```python
from build123d import *

# Parameters (mm, degrees)
EXTRUDE_1_DEPTH     = 10
HOLE_WIZARD_1_D     = 3.05
HOLE_WIZARD_1_DEPTH = 14
HOLE_WIZARD_2_D     = 5.01
HOLE_WIZARD_2_DEPTH = 14
HOLE_WIZARD_3_D     = 5.05
HOLE_WIZARD_3_DEPTH = 14
FILLET_1_R          = 2
FILLET_2_R          = 4


with BuildPart() as part:
    # 草图1 → 凸台-拉伸1 (new body)
    with BuildSketch(Plane.XZ):
        with BuildLine():
            Line((-28, -5.5), (-28, -12.193872478))
            ThreePointArc((-28, -12.193872478), (-26.845236523, -14.006488052), (-24.714424781, -13.725961365))
            Line((-24.714424781, -13.725961365), (-13.123475383, -4))
            Line((-13.123475383, -4), (-5.123475383, -4))
            ThreePointArc((-5.123475383, -4), (-0.488094847, -6.481648202), (4.466659496, -4.722176717))
            add(Edge.make_bspline(
                [(20.490071148, 0), (14.378134184, 3.89268165), (4.466659496, -4.722176717)],
                knots=[0.252803303, 0.252803303, 0.252803303, 2.064431363, 2.064431363, 2.064431363], degree=2, weights=[1, 0.617045201, 1]))
            ThreePointArc((20.490071148, 0), (24.593372298, 1.499185377), (22.849655998, 5.50469291))
            add(Edge.make_bspline(
                [(4.159420521, 4.994919512), (11.553776754, 7.153354998), (17.783855246, 7.323279465), (22.849655998, 5.50469291)],
                knots=[0, 0, 0, 0, 1, 1, 1, 1], degree=3))
            ThreePointArc((4.159420521, 4.994919512), (-0.692687991, 6.462985637), (-5.123475383, 4))
            Line((-5.123475383, 4), (-28.225082782, 4))
            ThreePointArc((-28.225082782, 4), (-37.111262075, 2.031009601), (-32, -5.5))
            Line((-32, -5.5), (-28, -5.5))
        make_face()
    extrude(amount=-EXTRUDE_1_DEPTH)

    # 草图2 → 旋转1 (revolve)
    with BuildSketch(Plane(origin=(0, 0, 0), x_dir=(-1, 0, 0), z_dir=(0, 0, -1)), mode=Mode.PRIVATE) as revolve_1_sk:
        Polygon((-3.99, -4), (0, -4), (0, 0), (-5, 0), (-5, -0.5), (-3.99, -0.5), align=None)
    revolve(revolve_1_sk.sketch.rotate(Axis((0, -4, 0), (0, 1, 0)), 270), axis=Axis((0, -4, 0), (0, 1, 0)))

    # 草图3 → 旋转2 (revolve)
    with BuildSketch(Plane.XY, mode=Mode.PRIVATE) as revolve_2_sk:
        Polygon((3.99, 14), (0, 14), (0, 10), (5, 10), (5, 10.5), (3.99, 10.5), align=None)
    revolve(revolve_2_sk.sketch.rotate(Axis((0, 14, 0), (0, -1, 0)), 270), axis=Axis((0, 14, 0), (0, -1, 0)))

    # 孔1
    with Locations(Plane(origin=(0, 10, 0), x_dir=(1, 0, 0), z_dir=(0, 1, 0))):
        with Locations((21.836015336, -2.681125555)):
            Hole(HOLE_WIZARD_1_D / 2, depth=HOLE_WIZARD_1_DEPTH)

    # 孔2
    with Locations(Plane(origin=(0, 10, 0), x_dir=(1, 0, 0), z_dir=(0, 1, 0))):
        with Locations((-23.339745962, 5)):
            Hole(HOLE_WIZARD_2_D / 2, depth=HOLE_WIZARD_2_DEPTH)

    # 孔3
    with Locations(Plane(origin=(0, 10, 0), x_dir=(1, 0, 0), z_dir=(0, 1, 0))):
        with Locations((-32, 0)):
            Hole(HOLE_WIZARD_3_D / 2, depth=HOLE_WIZARD_3_DEPTH)

    # 圆角1
    fillet_1_edges = [part.edges().sort_by_distance(p)[0] for p in [
        (-28, 5, -5.5),
    ]]
    fillet(fillet_1_edges, radius=FILLET_1_R)

    # 圆角2
    fillet_2_edges = [part.edges().sort_by_distance(p)[0] for p in [
        (-13.123475383, 5, -4),
    ]]
    fillet(fillet_2_edges, radius=FILLET_2_R)


solid = part.part
```
Part model, mm, in its own coordinate system. A direction names the side the tool comes from. Round coordinates to 2 decimals unless told otherwise and drop trailing zeros. Write each loop counter-clockwise with the first axis right and the second up, starting at its lowest first coordinate (ties: lowest second). Pieces come first, ordered by that corner, then holes. Notation, with made-up numbers: M -17,-27 L -8,-27 A23 cw -8,-10 Z; hole C 54.25,17.25 d1. An arc over 180 degrees is marked long. One line per question, with ' | ' between items.
(1) 3-axis set-ups, long thin cutter, end or side, ignore diameter. For faces 4 (the face through (-31, 5, -5.5)), 5 (the face through (-17, 5, 4)), 6 (the face through (-8, 5, -4)), 7 (the face through (-4, 10.5, 2)), 8 (the face through (-4, -0.5, -2)): which of +Z, -Z, +X, -X, +Y, -Y reach the whole face in a straight line?
Answer key:
face 4: -Z, -X, +Y, -Y | face 5: +Z, +Y, -Y | face 6: -Z, +Y, -Y | face 7: +Y | face 8: -Y
(2) Saw through at B-B on x = 0. Write the cut outline in (y, z), then the cut area to 3 significant figures.
Answer key:
outline: M -4,-3.99 L -0.5,-3.99 L -0.5,-5 L 0,-5 L 0,-6.5 L 10,-6.5 L 10,-5 L 10.5,-5 L 10.5,-3.99 L 14,-3.99 L 14,3.99 L 10.5,3.99 L 10.5,5 L 10,5 L 10,6.5 L 0,6.5 L 0,5 L -0.5,5 L -0.5,3.99 L -4,3.99 Z | area: 196 mm^2
(3) Two-plate mould, pull along Z, no slides. Class faces 1 (the face through (-22.797, 4.93, -2.555)), 2 (the face through (-0.564, 4.93, -6.476)), 3 (the face through (3.956, 12.274, 0.519)): released by +Z, released by -Z, zero draft, split by the parting line, or undercut.
Answer key:
face 1: undercut | face 2: released by -Z | face 3: split by the parting line
(4) Saw through at A-A on x = -22. Write the cut outline in (y, z).
Answer key:
outline: M 0,-11.45 L 10,-11.45 L 10,-7.12 L 0,-7.12 Z; M 0,-2.88 L 10,-2.88 L 10,4 L 0,4 Z
(5) Probe line 1 along Z through (x, y) = (-32, 4) (3 decimals); line 2 along X through (y, z) = (5, -4.5); line 3 along Y through (x, z) = (-27.5, 3.5). List the from-to ranges inside material, lowest first.
Answer key:
line 1: z = -5.5 to -2.525, 2.525 to 5.5 | line 2: x = -35.16 to -25.79, -20.89 to -13.6, -4.69 to 4.73 | line 3: y = 0 to 10
(6) Saw through at C-C on y = -2. Write the cut outline in (x, z).
Answer key:
outline: C 0,0 d7.98
(7) Pin check, flat tips, straight feed: pin 1 (4 mm diameter, centred on x = -25, y = 5, fed in from +Z); pin 2 (4.5 mm diameter, centred on x = -32, z = 0, fed in from -Y); pin 3 (5 mm diameter, centred on x = -8.5, y = 5.5, fed in from -Z); pin 4 (10 mm diameter, centred on x = -13, z = 4, fed in from +Y). Stop position of each tip, or through.
Answer key:
pin 1: stops at z = 4 | pin 2: passes through | pin 3: stops at z = -4 | pin 4: stops at y = 10
(8) Saw through at D-D on y = 9.25. Count the separate pieces of the cut face and the enclosed holes in it, then the cut area to 3 significant figures.
Answer key:
separate pieces: 1 | enclosed holes: 3 | area: 564 mm^2
